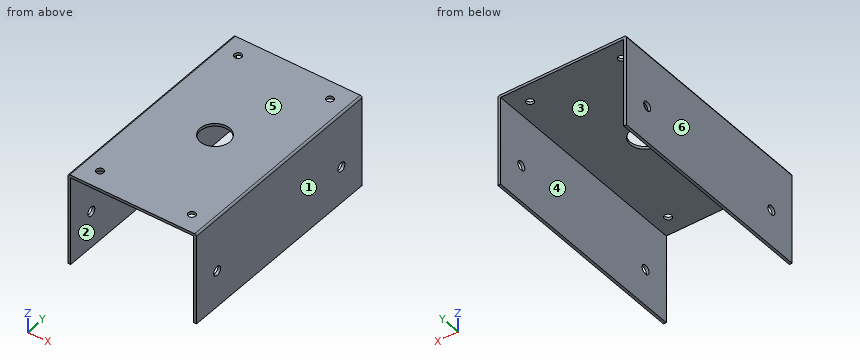
from build123d import *

# Parameters (mm, degrees)
EXTRUDE001_DEPTH                     = 120
EXTRUDE001_ONTO_SKETCH004_ROLL_ANGLE = 90
FILLET_R                             = 1
SKETCH005_R                          = 2.5
POCKET_DEPTH                         = 71
SKETCH007_R                          = 8
SKETCH007_R_2                        = 2
POCKET001_DEPTH                      = 5


with BuildPart() as part:
    # Sketch004 as drawn → Extrude001 (new)
    with BuildSketch(Plane.XY):
        Polygon((-35, 0), (-35, 50), (35, 50), (35, 0), (33.5, 0), (33.5, 48.5), (-33.5, 48.5), (-33.5, 0), align=None)
    extrude(amount=-EXTRUDE001_DEPTH)


with BuildPart() as part_1:
    # Extrude001 onto Sketch004 roll: moved
    add(part.part.rotate(Axis((0, 0, 0), (1, 0, 0)), EXTRUDE001_ONTO_SKETCH004_ROLL_ANGLE))


with BuildPart() as part_2:
    # Extrude001 onto Sketch004 placement: moved
    add(part_1.part)


with BuildPart() as part_3:
    # Extrude001 placement: moved
    add(part_2.part.moved(Location((0, -60, 0))))

    # Fillet
    fillet_edges = [part_3.edges().sort_by_distance(p)[0] for p in [
        (-35, 0, 50),
        (35, 0, 50),
    ]]
    fillet(fillet_edges, radius=FILLET_R)

    # Sketch005 → Pocket (cut)
    with BuildSketch(Plane.YZ.offset(35)):
        with Locations((-45, 20)):
            Circle(SKETCH005_R)
        with Locations((45, 20)):
            Circle(SKETCH005_R)
    extrude(amount=-POCKET_DEPTH, mode=Mode.SUBTRACT)

    # Sketch007 → Pocket001 (cut)
    with BuildSketch(Plane.XY.offset(50)):
        Circle(SKETCH007_R)
        with Locations((-25, 50)):
            Circle(SKETCH007_R_2)
        with Locations((25, 50)):
            Circle(SKETCH007_R_2)
        with Locations((-25, -50)):
            Circle(SKETCH007_R_2)
        with Locations((25, -50)):
            Circle(SKETCH007_R_2)
    extrude(amount=-POCKET001_DEPTH, mode=Mode.SUBTRACT)


solid = part_3.part
For this review, take the finished solid that the model builds, in its own axes (mm). Face numbers are marked on the shaded views. A direction names the side the tool comes from. Round coordinates to 2 decimals unless told otherwise and drop trailing zeros. Loops run counter-clockwise (first coordinate to the right, second up) from the corner with the lowest first, then second, coordinate; pieces in that order, holes last. Notation, with made-up numbers: (65, 45.5) - (124, 45.5) arc R13 cw to (124, 65.5) - close; hole circle Ø11 at (87.25, -17). An arc over 180 degrees is marked (long way). Use one line per item in the form item = value.
1) We need section C-C on z = 20. Write out the cut boundary in (x, y).
Solutions:
outline = (-35, -60) - (-33.5, -60) - (-33.5, -47.5) - (-35, -47.5) - close; (-35, -42.5) - (-33.5, -42.5) - (-33.5, 42.5) - (-35, 42.5) - close; (-35, 47.5) - (-33.5, 47.5) - (-33.5, 60) - (-35, 60) - close; (33.5, -60) - (35, -60) - (35, -47.5) - (33.5, -47.5) - close; (33.5, -42.5) - (35, -42.5) - (35, 42.5) - (33.5, 42.5) - close; (33.5, 47.5) - (35, 47.5) - (35, 60) - (33.5, 60) - close
2) We need section D-D on y = -45. Write out the cut boundary in (x, z).
Solutions:
outline = (-35, 0) - (-33.5, 0) - (-33.5, 17.5) - (-35, 17.5) - close; (-35, 22.5) - (-33.5, 22.5) - (-33.5, 48.5) - (33.5, 48.5) - (33.5, 22.5) - (35, 22.5) - (35, 49) arc R1 ccw to (34, 50) - (-34, 50) arc R1 ccw to (-35, 49) - close; (33.5, 0) - (35, 0) - (35, 17.5) - (33.5, 17.5) - close
3) Mouldability with a two-part tool opening along X and no side actions: class the marked faces 3, 4, 5 and 6 as pulls with the +X half, pulls with the -X half, needs draft (parallel to the pull), parting line crosses it, or undercut.
Solutions:
face_3 = undercut
face_4 = undercut
face_5 = needs draft
face_6 = pulls with the -X half
4) Tool access review of the marked faces 1 and 2: name each direction out of +Z, -Z, +X, -X, +Y, -Y from which nothing blocks a thin tool from reaching the whole face with its end or side.
Solutions:
face_1 = +Z, -Z, +X, +Y, -Y
face_2 = -Z, +Y, -Y
5) We need section B-B on y = 0. Write out the cut boundary in (x, z), then the cut area to 3 significant figures.
Solutions:
outline = (-35, 0) - (-33.5, 0) - (-33.5, 48.5) - (-8, 48.5) - (-8, 50) - (-34, 50) arc R1 ccw to (-35, 49) - close; (8, 48.5) - (33.5, 48.5) - (33.5, 0) - (35, 0) - (35, 49) arc R1 ccw to (34, 50) - (8, 50) - close
area = 226 mm2
6) We need section A-A on x = -25. Write out the cut boundary in (y, z), then the cut area to 3 significant figures.
Solutions:
outline = (-60, 48.5) - (-52, 48.5) - (-52, 50) - (-60, 50) - close; (-48, 48.5) - (48, 48.5) - (48, 50) - (-48, 50) - close; (52, 48.5) - (60, 48.5) - (60, 50) - (52, 50) - close
area = 168 mm2
7) Clearance check with flat-ended pins moving along their axes: P1, Ø4.5, axis at y = 45, z = 20, coming from the +X side; P2, Ø18.5, axis at x = 0, y = 0, coming from the -Z side. State where each tip first meets the part, or that it passes through.
Solutions:
P1 = through
P2 = 48.5
8) Wall thickness on probe 1 along Y at (x, z) = (25, 48.9); probe 2 along X at (y, z) = (52.5, 17); probe 3 along Z at (x, y) = (-7.5, -49): over which ranges is each line inside the solid? List them lowest first.
Solutions:
probe_1 = -60 to -52, -48 to 48, 52 to 60
probe_2 = -35 to -33.5, 33.5 to 35
probe_3 = 48.5 to 50
